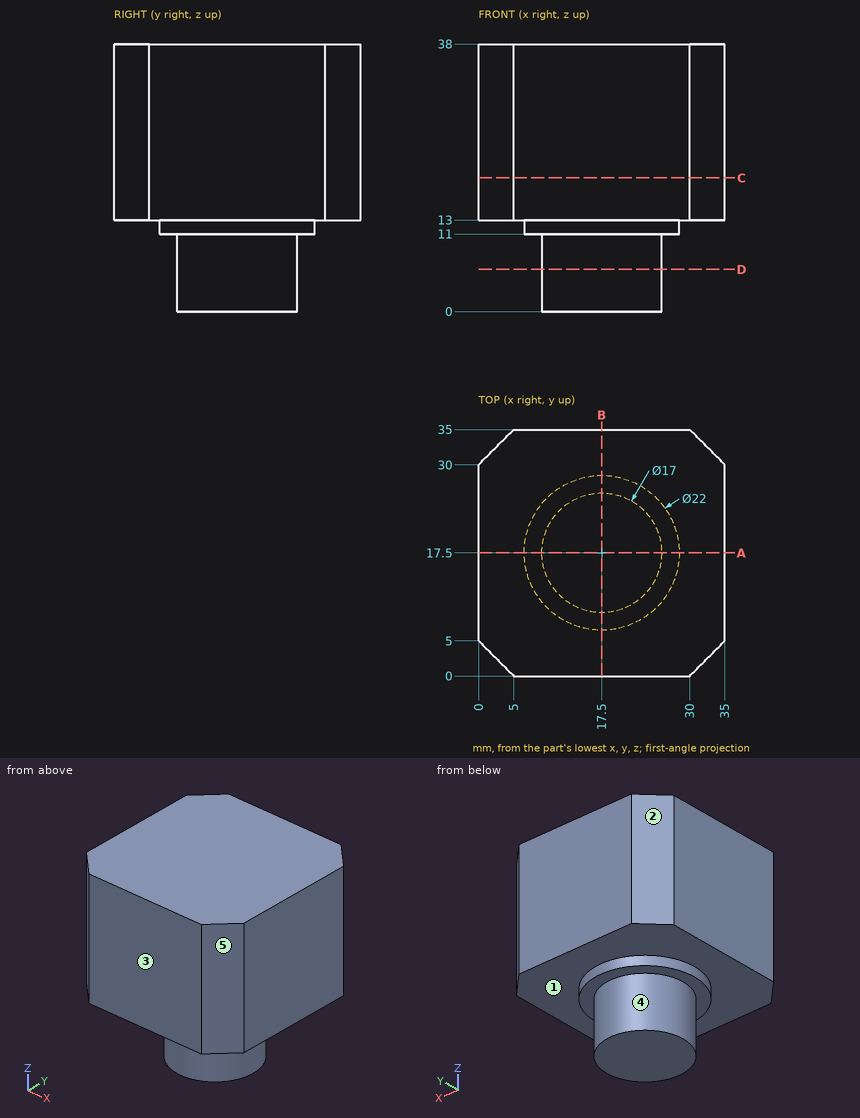
Answer from the drawing. Dimensions are ordinates in mm from the lowest x, y and z of the part. A direction names the side the tool comes from. Give positions to 0.01 mm unless a question says otherwise; leave off trailing zeros. Loops run counter-clockwise (first coordinate to the right, second up) from the corner with the lowest first, then second, coordinate; pieces in that order, holes last. Notation, with made-up numbers: (-12, 58.5) -> (-2, 58.5) arc R19 ccw to (-2, 70.5) -> close; hole circle Ø5 at (34, -39). An arc over 180 degrees is marked (long way). One line per question, with ' | ' between items. Start each with the question number.
1) Section D-D, the plane z = 6 is taken. Determine the outline of the cut face in (x, y).
2) Each of these flat-tipped pins is pushed along its axis until it touches: pin 1 (5 mm diameter, centred on x = 25.5, z = 9.5, fed in from -Y); pin 2 (2 mm diameter, centred on y = 7, z = 6, fed in from -X). Where does it stop, or does it pass through?
3) Section A-A, the plane y = 17.5 is taken. Determine the outline of the cut face in (x, z).
4) For the marked faces 1 and 2, determine the directions among +Z, -Z, +X, -X, +Y, -Y from which every point of the face is accessible in a straight line to the end or side of a thin tool.
5) Section C-C, the plane z = 19 is taken. Determine the outline of the cut face in (x, y), then the cut area to 4 significant figures.
6) Determine the mould class of the marked faces 3, 4 and 5 for opening direction X: +X half, -X half, draft (parallel to the pull), parting line (faces both ways), or undercut.
7) Straight lines are drawn through the part: L1, parallel to Z at x = 20, y = 4.5; L2, parallel to Y at x = 32.5, z = 22.5; L3, parallel to Y at x = 21, z = 5.5. For each, find the intervals that lie inside material, in ascending order.
Resolved:
1) outline: circle Ø17 at (17.5, 17.5)
2) pin 1: y = 8.28 | pin 2: through
3) outline: (0, 13) -> (6.5, 13) -> (6.5, 11) -> (9, 11) -> (9, 0) -> (26, 0) -> (26, 11) -> (28.5, 11) -> (28.5, 13) -> (35, 13) -> (35, 38) -> (0, 38) -> close
4) face 1: -Z | face 2: +Z, -Z, -X, +Y
5) outline: (0, 5) -> (5, 0) -> (30, 0) -> (35, 5) -> (35, 30) -> (30, 35) -> (5, 35) -> (0, 30) -> close | area: 1,175 mm2
6) face 3: draft | face 4: parting line | face 5: +X half
7) L1: 13 to 38 | L2: 2.5 to 32.5 | L3: 9.75 to 25.25
